Build history of the part. All positions in model axes, mm. A direction names the side the tool comes from. Round coordinates to 2 decimals unless told otherwise and drop trailing zeros. Order: outer loops, then holes, each group sorted by start corner. A loop starts at its lowest first (then second) coordinate and runs counter-clockwise, first axis right, second up. Notation, with made-up numbers: (10.25, 77.25) -> (36.25, 77.25) arc R15 cw to (36.25, 104.25) -> close; hole circle Ø5 at (49, 74). An arc over 180 degrees is marked (long way). Answer as a JSON object with one key per item and string values.
from build123d import *

# Parameters (mm, degrees)
ESQUISSE2_R        = 3.25
BOSS_EXTRU_1_DEPTH = 3
CONG_1_R           = 5


with BuildPart() as part:
    # Esquisse2 → Boss.-Extru.1 (new body)
    with BuildSketch(Plane.XY):
        Polygon((107.208492459, 1.901473412), (39.208492459, 1.901473412), (39.208492459, -43.098526588), (55.708492459, -43.098526588), (55.708492459, -58.098526588), (90.708492459, -58.098526588), (90.708492459, -43.098526588), (107.208492459, -43.098526588), align=None)
        with Locations((102.208492459, -4.098526588)):
            Circle(ESQUISSE2_R, mode=Mode.SUBTRACT)
        with Locations((102.208492459, -38.098526588)):
            Circle(ESQUISSE2_R, mode=Mode.SUBTRACT)
        with Locations((44.208492459, -38.098526588)):
            Circle(ESQUISSE2_R, mode=Mode.SUBTRACT)
        with Locations((44.208492459, -4.098526588)):
            Circle(ESQUISSE2_R, mode=Mode.SUBTRACT)
        with Locations((44.208492459, -21.098526588)):
            Circle(ESQUISSE2_R, mode=Mode.SUBTRACT)
        with Locations((102.208492459, -21.098526588)):
            Circle(ESQUISSE2_R, mode=Mode.SUBTRACT)
    extrude(amount=BOSS_EXTRU_1_DEPTH)

    # Congé1
    cong_1_edges = [part.edges().sort_by_distance(p)[0] for p in [
        (107.208492459, -43.098526588, 1.5),
        (90.708492459, -43.098526588, 1.5),
        (90.708492459, -58.098526588, 1.5),
        (55.708492459, -58.098526588, 1.5),
        (55.708492459, -43.098526588, 1.5),
        (39.208492459, -43.098526588, 1.5),
        (39.208492459, 1.901473412, 1.5),
        (107.208492459, 1.901473412, 1.5),
    ]]
    fillet(cong_1_edges, radius=CONG_1_R)


solid = part.part
1) Cut at A-A, the plane y = -5. Give the cut face in (x, z).
Checked values:
{"outline": "(39.21, 0) -> (41.09, 0) -> (41.09, 3) -> (39.21, 3) -> close; (47.33, 0) -> (99.09, 0) -> (99.09, 3) -> (47.33, 3) -> close; (105.33, 0) -> (107.21, 0) -> (107.21, 3) -> (105.33, 3) -> close"}
2) Cut at C-C, the plane y = -44. Give the cut face in (x, z).
Checked values:
{"outline": "(53.57, 0) -> (92.84, 0) -> (92.84, 3) -> (53.57, 3) -> close"}
3) Probe L1, parallel to Y at x = 101.5, z = 2; L2, parallel to X at y = -7, z = 2; L3, parallel to X at y = -35.5, z = 0.2. List the from-to ranges inside material, lowest first. Write a range as from..to.
Checked values:
{"L1": "y = -43.1..-41.27, -34.93..-24.27, -17.93..-7.27, -0.93..1.9", "L2": "x = 39.21..42.74, 45.67..100.74, 103.67..107.21", "L3": "x = 39.21..42.26, 46.16..100.26, 104.16..107.21"}
4) Cut at B-B, the plane z = 0.6. Give the cut face in (x, y).
Checked values:
{"outline": "(39.21, -38.1) arc R5 ccw to (44.21, -43.1) -> (50.71, -43.1) arc R5 cw to (55.71, -48.1) -> (55.71, -53.1) arc R5 ccw to (60.71, -58.1) -> (85.71, -58.1) arc R5 ccw to (90.71, -53.1) -> (90.71, -48.1) arc R5 cw to (95.71, -43.1) -> (102.21, -43.1) arc R5 ccw to (107.21, -38.1) -> (107.21, -3.1) arc R5 ccw to (102.21, 1.9) -> (44.21, 1.9) arc R5 ccw to (39.21, -3.1) -> close; hole circle Ø6.5 at (44.21, -38.1); hole circle Ø6.5 at (44.21, -21.1); hole circle Ø6.5 at (44.21, -4.1); hole circle Ø6.5 at (102.21, -38.1); hole circle Ø6.5 at (102.21, -21.1); hole circle Ø6.5 at (102.21, -4.1)"}
5) Flat gauge pins, fed straight in: pin 1 Ø1.5 at (y, z) = (-44.5, 1) entering from -X; pin 2 Ø1.5 at (y, z) = (-49.5, 2) entering from -X; pin 3 Ø0.9 at (y, z) = (-50, 1) entering from +X. Where does each tip first touch, or does it go through?
Checked values:
{"pin 1": "stops at x = 53.18", "pin 2": "stops at x = 55.71", "pin 3": "stops at x = 90.71"}
6) Pull direction Y, two halves, no side cores. Call faces 1 (the face through (105.7, 0.48, 1.52)), 2 (the face through (99, -43.099, 1)), 3 (the face through (105.3, -3.1, 1.5)): pulls with the +Y half, pulls with the -Y half, needs draft (parallel to the pull), parting line crosses it, or undercut.
Checked values:
{"face 1": "pulls with the +Y half", "face 2": "pulls with the -Y half", "face 3": "undercut"}
7) Which spindle directions (+Z, -Z, +X, -X, +Y, -Y) get a long thin tool onto all of the face, cutting with end or side? Do faces 4 (the face through (55.708, -51, 1)), 5 (the face through (90.708, -51, 1)), 6 (the face through (73, -28, 3)). Say none if no direction does.
Checked values:
{"face 4": "+Z, -Z, -X, -Y", "face 5": "+Z, -Z, +X, -Y", "face 6": "+Z, +X, -X, +Y, -Y"}
